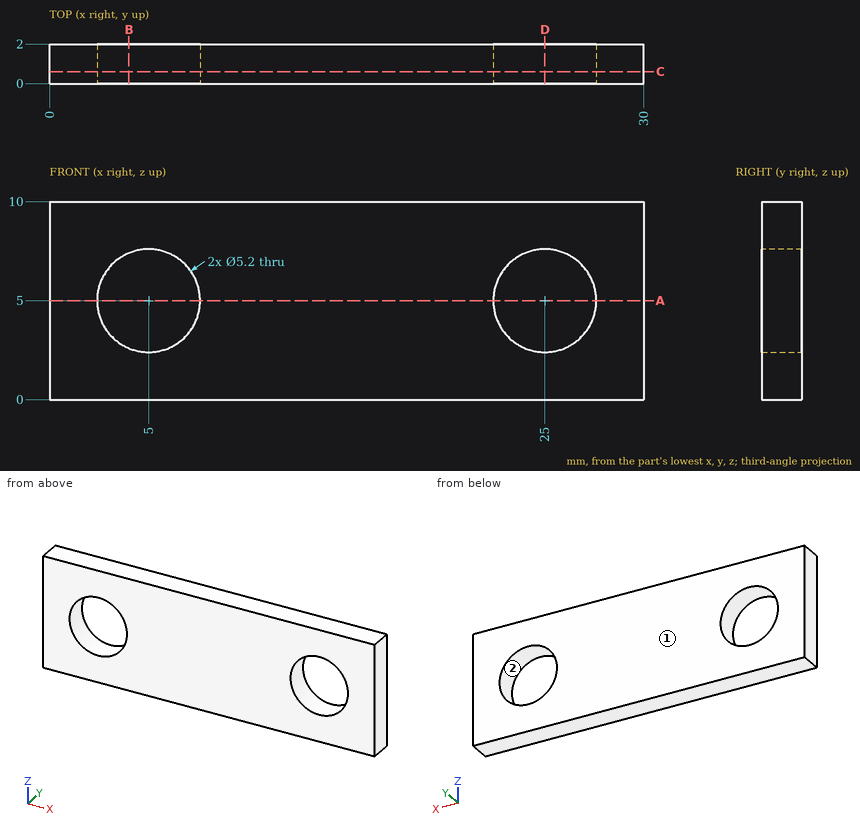
Answer from the drawing. Dimensions are ordinates in mm from the lowest x, y and z of the part. Round coordinates to 2 decimals unless told otherwise and drop trailing zeros. Write each loop counter-clockwise with the first axis right and the second up, starting at its lowest first coordinate (ties: lowest second). Pieces come first, ordered by that corner, then holes. Notation, with made-up numbers: (4, 70) - (54, 70) arc R19 ccw to (54, 102) - close; hole circle Ø10 at (71, 34.25). An arc over 180 degrees is marked (long way). One line per item, written item: value.
Q1. Straight lines are drawn through the part: line 1 (X direction, y = 0.65, z = 5); line 2 (X direction, y = 0.1, z = 5.75); line 3 (Z direction, x = 27.25, y = 0.9). For each, find the intervals that lie inside material, in ascending order. Write a range as from..to.
The answers:
line 1: x = 0..2.4, 7.6..22.4, 27.6..30
line 2: x = 0..2.51, 7.49..22.51, 27.49..30
line 3: z = 0..3.7, 6.3..10
Q2. Find section B-B (x = 4). Determine the outline of the cut face in (y, z), and give its area (3 significant figures).
The answers:
outline: (0, 0) - (2, 0) - (2, 2.6) - (0, 2.6) - close; (0, 7.4) - (2, 7.4) - (2, 10) - (0, 10) - close
area: 10.4 mm2
Q3. For a pull along Z with two mould halves and no side action, classify the marked faces 1 and 2 as pulls with the +Z half, pulls with the -Z half, needs draft (parallel to the pull), parting line crosses it, or undercut.
The answers:
face 1: needs draft
face 2: undercut
Q4. Find section D-D (x = 25). Determine the outline of the cut face in (y, z).
The answers:
outline: (0, 0) - (2, 0) - (2, 2.4) - (0, 2.4) - close; (0, 7.6) - (2, 7.6) - (2, 10) - (0, 10) - close
Q5. Find section A-A (z = 5). Determine the outline of the cut face in (x, y).
The answers:
outline: (0, 0) - (2.4, 0) - (2.4, 2) - (0, 2) - close; (7.6, 0) - (22.4, 0) - (22.4, 2) - (7.6, 2) - close; (27.6, 0) - (30, 0) - (30, 2) - (27.6, 2) - close
Q6. This flat-tipped pin is pushed along its axis until it touches: P1, Ø2, axis at x = 23.5, z = 2.5, coming from the -Y side. Where does it stop, or does it pass through?
The answers:
P1: stops at y = 0
Q7. Find section C-C (y = 0.6). Determine the outline of the cut face in (x, z), and give its area (3 significant figures).
The answers:
outline: (0, 0) - (30, 0) - (30, 10) - (0, 10) - close; hole circle Ø5.2 at (5, 5); hole circle Ø5.2 at (25, 5)
area: 258 mm2
